```python
from build123d import *

# Parameters (mm, degrees)
SKETCH_W     = 10
SKETCH_H     = 25
PAD_DEPTH    = 5
CHAMFER_SIZE = 4


with BuildPart() as part:
    # Sketch → Pad (new body)
    with BuildSketch(Plane.XZ):
        Polygon((-50, -35), (50, -25), (50, 25), (-50, 35), align=None)
        with Locations((25, 0)):
            Rectangle(SKETCH_W, SKETCH_H, mode=Mode.SUBTRACT)
    extrude(amount=PAD_DEPTH)

    # Chamfer
    chamfer_edges = [part.edges().sort_by_distance(p)[0] for p in [
        (0, 0, 30),
        (50, 0, 0),
        (0, 0, -30),
        (-50, 0, 0),
    ]]
    chamfer(chamfer_edges, length=CHAMFER_SIZE)


solid = part.part
```
Here's how the part is built. I have some questions about the finished solid (model axes, mm). A direction names the side the tool comes from. Round coordinates to 2 decimals unless told otherwise and drop trailing zeros. Order: outer loops, then holes, each group sorted by start corner. A loop starts at its lowest first (then second) coordinate and runs counter-clockwise, first axis right, second up. Notation, with made-up numbers: M -17.5,15.25 L -6.5,15.25 A5 ccw -6.5,23.25 Z; hole C 56.5,12 d3. An arc over 180 degrees is marked long. Answer in a Markdown table with one row per item.
Item 1: Imagine slicing it at C-C, the plane x = 8.5. Write out the boundary of the cut face in (y, z).
A:
| item | result |
|---|---|
| outline | M -5,-29.15 L -4,-29.15 L 0,-25.13 L 0,25.13 L -4,29.15 L -5,29.15 Z |
Item 2: If I drill on L1, parallel to Z at x = 29.5, y = -1.3; L2, parallel to Z at x = 23, y = -1.65; L3, parallel to X at y = -1.8, z = 0, over which ranges is the centre line in solid material (lowest first)? Write a range as from..to.
A:
| item | result |
|---|---|
| L1 | z = -24.34..-12.5, 12.5..24.34 |
| L2 | z = -25.34..-12.5, 12.5..25.34 |
| L3 | x = -47.8..20, 30..47.8 |
Item 3: Thinking about a two-plate mould opening in X: for faces 1 (the face through (30, -2, 0)), 2 (the face through (-48, -2, 0)), 3 (the face through (-1, -5, 0)), 4 (the face through (-0.9, -1.97, -28.05)), which applies, +X half, -X half, draft (parallel to the pull), parting line (faces both ways), or undercut?
A:
| item | result |
|---|---|
| face 1 | undercut |
| face 2 | -X half |
| face 3 | draft |
| face 4 | +X half |
Item 4: Imagine slicing it at B-B, the plane z = 20. Write out the boundary of the cut face in (x, y).
A:
| item | result |
|---|---|
| outline | M -50,-5 L 50,-5 L 50,-4 L 46,0 L -46,0 L -50,-4 Z |
Item 5: For faces 5 (the face through (0.7, -4.49, 29.93)), 6 (the face through (20, -2, 0)), which set-ups out of +Z, -Z, +X, -X, +Y, -Y let a thin tool reach every point of the face, with its end or its side?
A:
| item | result |
|---|---|
| face 5 | +Z, +X, +Y, -Y |
| face 6 | +Y, -Y |
Item 6: I'm going to push flat-ended pins straight in: pin 1 (2 mm diameter, centred on y = -1.5, z = -7.5, fed in from +X); pin 2 (1.5 mm diameter, centred on x = 27, y = -2, fed in from -Z); pin 3 (1.5 mm diameter, centred on x = 5, y = -4, fed in from -Z) (3 decimals). Where does each tip first touch, or does it pass through?
A:
| item | result |
|---|---|
| pin 1 | stops at x = 48.5 |
| pin 2 | stops at z = -26.05 |
| pin 3 | stops at z = -29.575 |
Item 7: Imagine slicing it at A-A, the plane y = -1.35. Write out the boundary of the cut face in (x, z).
A:
| item | result |
|---|---|
| outline | M -47.35,-32.07 L 47.35,-22.6 L 47.35,22.6 L -47.35,32.07 Z; hole M 20,-12.5 L 30,-12.5 L 30,12.5 L 20,12.5 Z |
